Could you check a few things on this model? Use its own coordinates, in mm. Give positions to 0.01 mm unless a question says otherwise; leave off trailing zeros. Loops run counter-clockwise (first coordinate to the right, second up) from the corner with the lowest first, then second, coordinate; pieces in that order, holes last. Notation, with made-up numbers: (16, -22.5) -> (41, -22.5) arc R15 cw to (41, -11.5) -> close; hole circle Ø7 at (8.25, -16.75). An arc over 180 degrees is marked (long way). Put each result on its own line as item: value.
```python
from build123d import *

# Parameters (mm, degrees)
F0_R     = 2.62001
F0_R_2   = 2.55651
F1_DEPTH = 9.525
F3_DEPTH = 1.7719311324


with BuildPart() as f1:
    # F0 (on Top) → F1 (new body)
    with BuildSketch(Plane.XY):
        with BuildLine():
            Line((0, 8.128), (0, 0))
            Line((0, 0), (12.5984, 0))
            ThreePointArc((12.5984, 0), (16.6624, 4.064), (12.5984, 8.128))
            Line((12.5984, 8.128), (0, 8.128))
        make_face()
        with Locations((3.9624, 4.064)):
            Circle(F0_R, mode=Mode.SUBTRACT)
        with Locations((12.5984, 4.064)):
            Circle(F0_R_2, mode=Mode.SUBTRACT)
    extrude(amount=F1_DEPTH)

    # F2 (on face) → F3 (cut, through all)
    with BuildSketch(Plane.XZ):
        with BuildLine():
            Line((12.5984, 3.6322), (12.5984, 5.8928))
            ThreePointArc((12.5984, 5.8928), (11.4681, 4.7625), (12.5984, 3.6322))
        make_face()
        with BuildLine():
            ThreePointArc((12.5984, 3.6322), (13.3976427948, 3.9632572052), (13.7287, 4.7625))
            ThreePointArc((13.7287, 4.7625), (13.3976427948, 5.5617427948), (12.5984, 5.8928))
            Line((12.5984, 5.8928), (12.5984, 3.6322))
        make_face()
    extrude(amount=-F3_DEPTH, mode=Mode.SUBTRACT)


solid = f1.part
```
1. I need wall thicknesses on line 1 (X direction, y = 4, z = 2.5); line 2 (X direction, y = 2.75, z = 6.75); line 3 (Y direction, x = 3.5, z = 3). Which ranges of each line are inside material? Lowest first, please.
Recorded:
line 1: x = 0 to 1.34, 6.58 to 10.04, 15.15 to 16.66
line 2: x = 0 to 1.7, 6.23 to 10.41, 14.79 to 16.44
line 3: y = 0 to 1.49, 6.64 to 8.13
2. If we section it at B-B (x = 4): List the corners of the cut face in (y, z) for me (3 decimals), then the cut area to 3 significant figures.
Recorded:
outline: (0, 0) -> (1.444, 0) -> (1.444, 9.525) -> (0, 9.525) -> close; (6.684, 0) -> (8.128, 0) -> (8.128, 9.525) -> (6.684, 9.525) -> close
area: 27.5 mm^2
3. If we section it at A-A (y = 5.25): List the corners of the cut face in (x, z) for me (1 decimal), then the cut area to 3 significant figures.
Recorded:
outline: (0, 0) -> (1.6, 0) -> (1.6, 9.5) -> (0, 9.5) -> close; (6.3, 0) -> (10.3, 0) -> (10.3, 9.5) -> (6.3, 9.5) -> close; (14.9, 0) -> (16.5, 0) -> (16.5, 9.5) -> (14.9, 9.5) -> close
area: 69.4 mm^2
4. I'm going to push a flat-ended pin straight in: pin 1 (4.5 mm diameter, centred on x = 12.6, y = 4.06, fed in from +Z). Where does the tip first touch, or does it pass through?
Recorded:
pin 1: passes through
5. If we section it at C-C (z = 4.25): List the corners of the cut face in (x, y) for me.
Recorded:
outline: (0, 0) -> (11.59, 0) -> (11.59, 1.71) arc R2.56 cw (long way) to (13.61, 1.71) -> (13.61, 0.13) arc R4.06 ccw to (12.6, 8.13) -> (0, 8.13) -> close; hole circle Ø5.24 at (3.96, 4.06)
6. If we section it at D-D (y = 2.25): List the corners of the cut face in (x, z) for me (3 decimals), then the cut area to 3 significant figures.
Recorded:
outline: (0, 0) -> (2.072, 0) -> (2.072, 9.525) -> (0, 9.525) -> close; (5.853, 0) -> (10.797, 0) -> (10.797, 9.525) -> (5.853, 9.525) -> close; (14.4, 0) -> (16.235, 0) -> (16.235, 9.525) -> (14.4, 9.525) -> close
area: 84.3 mm^2
